Answer from the drawing. Dimensions are ordinates in mm from the lowest x, y and z of the part. A direction names the side the tool comes from. Give positions to 0.01 mm unless a question says otherwise; leave off trailing zeros. Loops run counter-clockwise (first coordinate to the right, second up) from the corner with the lowest first, then second, coordinate; pieces in that order, holes last. Notation, with made-up numbers: (49.5, -4) - (99.5, -4) arc R18 cw to (99.5, 1) - close; hole circle Ø1 at (19, -24.5). An arc over 180 degrees is marked (long way). Answer as CSV lines item,"result". Start each with the question number.
1) Flat-ended cylindrical pins translate along their axes: pin 1 (0.6 mm diameter, centred on x = 82, y = 1, fed in from +Z) (3 decimals); pin 2 (2.5 mm diameter, centred on x = 3, z = 12.5, fed in from +Y); pin 3 (0.6 mm diameter, centred on x = 83.5, y = 0.5, fed in from -Z) (3 decimals). Find the tip coordinate at first contact, or state that the pin passes through.
2) For the marked faces 1 and 2, determine the directions among +Z, -Z, +X, -X, +Y, -Y from which every point of the face is accessible in a straight line to the end or side of a thin tool.
3) A cutting plane is placed at B-B (z = 43.5). Determine the outline of the cut face in (x, y).
4) Find the intervals of material crossed by line 1 along X through (y, z) = (1.2, 20); line 2 along X through (y, z) = (0.45, 14); line 3 along X through (y, z) = (1.5, 31.5), in increasing order.
5) A cutting plane is placed at A-A (y = 1.3). Determine the outline of the cut face in (x, z) (3 decimals).
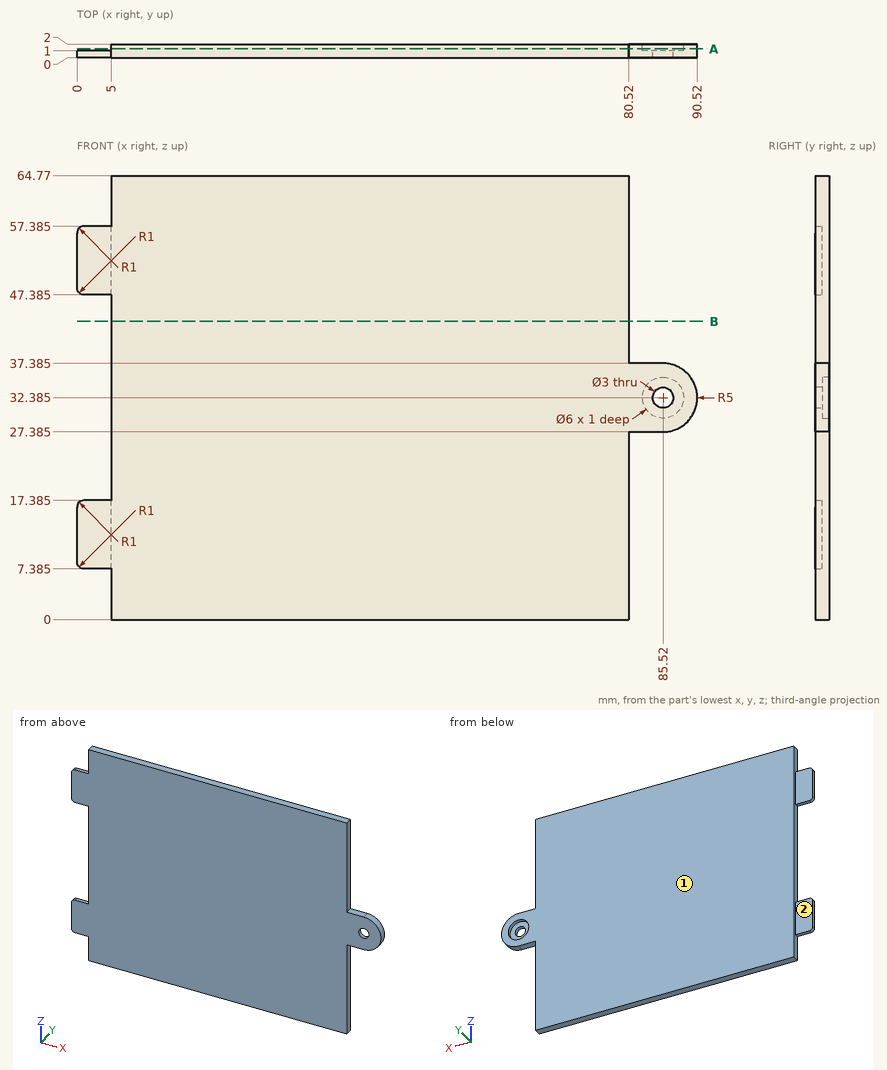
Ans:
1,pin 1,"z = 37.385"
1,pin 2,"y = 1"
1,pin 3,"z = 27.385"
2,face 1,"+Z, -Z, +X, -X, +Y"
2,face 2,"+Z, -Z, -X, +Y"
3,outline,"(5, 0) - (80.52, 0) - (80.52, 2) - (5, 2) - close"
4,line 1,"5 to 80.52"
4,line 2,"0 to 80.52"
4,line 3,"5 to 82.65, 88.39 to 90.44"
5,outline,"(5, 0) - (80.52, 0) - (80.52, 27.385) - (85.52, 27.385) arc R5 ccw to (85.52, 37.385) - (80.52, 37.385) - (80.52, 64.77) - (5, 64.77) - close; hole circle Ø6 at (85.52, 32.385)"
